```python
from build123d import *

# Parameters (mm, degrees)
SKETCH1_W           = 20
SKETCH1_H           = 20
BOSS_EXTRUDE1_DEPTH = 20
SKETCH2_W           = 20
SKETCH2_H           = 40.2
BOSS_EXTRUDE2_DEPTH = 64.7
SKETCH3_W           = 40.9
SKETCH3_H           = 20.8
CUT_EXTRUDE1_DEPTH  = 90.320210479
SKETCH4_W           = 11.9
SKETCH4_H           = 40.2
CUT_EXTRUDE2_DEPTH  = 90.320210479
SKETCH5_R           = 2.35
CUT_EXTRUDE3_DEPTH  = 10
SKETCH6_R           = 2.35
CUT_EXTRUDE4_DEPTH  = 10
CHAMFER1_SIZE       = 1
SKETCH7_W           = 20
SKETCH7_H           = 10.1
BOSS_EXTRUDE4_DEPTH = 4.7
SKETCH9_W           = 20
SKETCH9_H           = 20
BOSS_EXTRUDE5_DEPTH = 24.7
SKETCH10_R          = 3
CUT_EXTRUDE5_DEPTH  = 2
FILLET1_R           = 3.23
SKETCH11_W          = 20.2
SKETCH11_H          = 20.2
SKETCH11_W_2        = 20
SKETCH11_H_2        = 20
BOSS_EXTRUDE6_DEPTH = 40
SKETCH12_R          = 3.35
BOSS_EXTRUDE7_DEPTH = 0.1
BOSS_EXTRUDE8_DEPTH = 0.1


with BuildPart() as part:
    # Sketch1 → Boss-Extrude1 (new body)
    with BuildSketch(Plane(origin=(0, 0, 0), x_dir=(0, 0, -1), z_dir=(1, 0, 0))):
        Rectangle(SKETCH1_W, SKETCH1_H)
    extrude(amount=BOSS_EXTRUDE1_DEPTH)

    # Sketch2 → Boss-Extrude2 (add)
    with BuildSketch(Plane(origin=(20, 0, 0), x_dir=(0, 0, -1), z_dir=(1, 0, 0))):
        Rectangle(SKETCH2_W, SKETCH2_H)
    extrude(amount=BOSS_EXTRUDE2_DEPTH)

    # Sketch3 → Cut-Extrude1 (cut, through all)
    with BuildSketch(Plane.XY.offset(10)):
        with Locations((52.35, 0)):
            Rectangle(SKETCH3_W, SKETCH3_H)
    extrude(amount=-CUT_EXTRUDE1_DEPTH, mode=Mode.SUBTRACT)

    # Sketch4 → Cut-Extrude2 (cut, through all)
    with BuildSketch(Plane.XY.offset(10)):
        with Locations((78.75, 0)):
            Rectangle(SKETCH4_W, SKETCH4_H)
    extrude(amount=-CUT_EXTRUDE2_DEPTH, mode=Mode.SUBTRACT)

    # Sketch5 → Cut-Extrude3 (cut)
    with BuildSketch(Plane.XY.offset(10)):
        with Locations((28.01, 4.9)):
            Circle(SKETCH5_R)
        with Locations(Location((28.01, -4.9, 0), (0, 0, 180))):
            Circle(SKETCH5_R)
    extrude(amount=-CUT_EXTRUDE3_DEPTH, mode=Mode.SUBTRACT)

    # Sketch6 → Cut-Extrude4 (cut)
    with BuildSketch(Plane(origin=(72.8, 0, 0), x_dir=(0, 0, -1), z_dir=(1, 0, 0))):
        with Locations((0, -15.25)):
            Circle(SKETCH6_R)
        with Locations(Location((0, 15.25, 0), (0, 0, 180))):
            Circle(SKETCH6_R)
    extrude(amount=-CUT_EXTRUDE4_DEPTH, mode=Mode.SUBTRACT)

    # Chamfer1
    chamfer1_edges = [part.edges().sort_by_distance(p)[0] for p in [
        (25.66, 4.9, 10),
        (30.36, -4.9, 10),
        (72.8, -15.25, 2.35),
        (72.8, 15.25, -2.35),
    ]]
    chamfer(chamfer1_edges, length=CHAMFER1_SIZE)

    # Sketch7 → Boss-Extrude4 (add)
    with BuildSketch(Plane.ZY.offset(-20)):
        with Locations((0, 15.05)):
            Rectangle(SKETCH7_W, SKETCH7_H)
        with Locations((0, -15.05)):
            Rectangle(SKETCH7_W, SKETCH7_H)
    extrude(amount=BOSS_EXTRUDE4_DEPTH)

    # Sketch9 → Boss-Extrude5 (add)
    with BuildSketch(Plane.ZY):
        Rectangle(SKETCH9_W, SKETCH9_H)
    extrude(amount=BOSS_EXTRUDE5_DEPTH)

    # Sketch10 → Cut-Extrude5 (cut)
    with BuildSketch(Plane.ZY.offset(24.7)):
        Circle(SKETCH10_R)
    extrude(amount=-CUT_EXTRUDE5_DEPTH, mode=Mode.SUBTRACT)

    # Fillet1
    # the kernel refuses this fillet: 3.23 mm, written as the material it adds along each edge
    with BuildSketch(Plane(origin=(-22.7, 0, 0), x_dir=(0, 0, 1), z_dir=(0, -1, 0))) as fillet1_piece_1:
        with BuildLine():
            CenterArc((0.013363095, 3.23), FILLET1_R, 270, 67.616447755)
            Line((0.013363095, 0), (0.013363095, -0.0646))
            Line((0.013363095, -0.0646), (3, -0.0646))
            Line((3, -0.0646), (3.0646, 0))
            ThreePointArc((3.0646, 0), (3.0646, 1), (3.059732738, 1.9754))
            Line((3.059732738, 1.9754), (3, 2))
        make_face()
    revolve(axis=Axis((-22.7, 0, 0), (-1, 0, 0)))

    # Sketch11 → Boss-Extrude6 (add)
    with BuildSketch(Plane.ZY.offset(24.7)):
        Rectangle(SKETCH11_W, SKETCH11_H)
        Rectangle(SKETCH11_W_2, SKETCH11_H_2, mode=Mode.SUBTRACT)
    extrude(amount=-BOSS_EXTRUDE6_DEPTH)

    # Sketch12 → Boss-Extrude7 (add)
    with BuildSketch(Plane.XY.offset(10)):
        Polygon((72.8, 20.1), (15.3, 20.1), (15.3, -20.1), (72.8, -20.1), (72.8, -10.4), (31.9, -10.4), (31.9, 10.4), (72.8, 10.4), align=None)
        with Locations(Location((28.01, 4.9, 0), (0, 0, 180))):
            Circle(SKETCH12_R, mode=Mode.SUBTRACT)
        with Locations(Location((28.01, -4.9, 0), (0, 0, 180))):
            Circle(SKETCH12_R, mode=Mode.SUBTRACT)
    extrude(amount=BOSS_EXTRUDE7_DEPTH)

    # Sketch13 → Boss-Extrude8 (add)
    with BuildSketch(Plane(origin=(0, 0, -10), x_dir=(-1, 0, 0), z_dir=(0, 0, -1))):
        Polygon((-72.8, -20.1), (-15.3, -20.1), (-15.3, 20.1), (-72.8, 20.1), (-72.8, 10.4), (-31.9, 10.4), (-31.9, -10.4), (-72.8, -10.4), align=None)
    extrude(amount=BOSS_EXTRUDE8_DEPTH)


solid = part.part
```
Input: part model. Units: mm. Frame: model coordinates. A direction names the side the tool comes from. Give positions to 0.01 mm unless a question says otherwise; leave off trailing zeros. Write each loop counter-clockwise with the first axis right and the second up, starting at its lowest first coordinate (ties: lowest second). Pieces come first, ordered by that corner, then holes. Notation, with made-up numbers: (7, -12) - (61, -12) arc R11 cw to (61, -3) - close; hole circle Ø6 at (16.25, 12). An arc over 180 degrees is marked (long way). Write item = value, one per line. Start each with the question number.
1. Access query for faces 1 (the flat face through (62.8, 15, 0)), 2 (the flat face through (53, 10.4, 0)), 3 (the flat face through (28, -5, 0)), 4 (the flat face through (-5, 10.1, 0)). Directions: +Z, -Z, +X, -X, +Y, -Y. A direction counts if a zero-diameter tool reaches every point of the face in a straight line with its end or side. Return the directions, or none.
2. Section query D-D, the plane x = 28.01. Output: boundary loops of the cut face in (y, z).
3. Mould query, pull axis X, two halves, no side actions, for faces 5 (the flat face through (31.9, 0, 0)), 6 (the cylindrical face through (67.363, -17.544, 0.509)), 7 (the cylindrical face through (29.875, -3.47, 4.563)). Classes: released by +X, released by -X, zero draft, split by the parting line, or undercut.
4. Section query C-C, the plane z = -6. Output: boundary loops of the cut face in (x, y).
5. Section query A-A, the plane x = 60. Output: boundary loops of the cut face in (y, z).
6. Section query B-B, the plane y = -4.9. Output: boundary loops of the cut face in (x, z), then the cut area to 3 significant figures.
7. First-contact query: pin 1 Ø3 at (y, z) = (15.25, 0) entering from -X; pin 2 Ø10 at (x, z) = (2, 2.5) entering from +Y; pin 3 Ø1.4 at (y, z) = (16, 1) entering from +X; pin 4 Ø1.5 at (x, y) = (-12.5, 12.5) entering from -Z. Flat tips, straight axial feed; report the tip coordinate or a pass-through.
8. Ray query, L1, parallel to Y at x = 67.75, z = 0; L2, parallel to Y at x = 28.01, z = 2.75; L3, parallel to Y at x = 63, z = 8. Return the intervals inside material, ascending.
Check sheet entries:
q1.face_1 = +X
q1.face_2 = +Z, -Z, +X
q1.face_3 = +Z
q1.face_4 = +Z, -Z, -X, +Y
q2.outline = (-20.1, -10.1) - (20.1, -10.1) - (20.1, 10.1) - (8.25, 10.1) - (8.25, 10) - (7.25, 9) - (7.25, 0) - (2.55, 0) - (2.55, 9) - (1.55, 10) - (1.55, 10.1) - (-1.55, 10.1) - (-1.55, 10) - (-2.55, 9) - (-2.55, 0) - (-7.25, 0) - (-7.25, 9) - (-8.25, 10) - (-8.25, 10.1) - (-20.1, 10.1) - close
q3.face_5 = released by +X
q3.face_6 = zero draft
q3.face_7 = undercut
q4.outline = (-24.7, -10.1) - (15.3, -10.1) - (15.3, -20.1) - (72.8, -20.1) - (72.8, -10.4) - (31.9, -10.4) - (31.9, 10.4) - (72.8, 10.4) - (72.8, 20.1) - (15.3, 20.1) - (15.3, 10.1) - (-24.7, 10.1) - close
q5.outline = (-20.1, -10.1) - (-10.4, -10.1) - (-10.4, 10.1) - (-20.1, 10.1) - close; (10.4, -10.1) - (20.1, -10.1) - (20.1, 10.1) - (10.4, 10.1) - close
q6.outline = (-24.7, -10.1) - (31.9, -10.1) - (31.9, 10.1) - (31.36, 10.1) - (31.36, 10) - (30.36, 9) - (30.36, 0) - (25.66, 0) - (25.66, 9) - (24.66, 10) - (24.66, 10.1) - (-24.7, 10.1) - close
q6.area = 1,090 mm2
q7.pin_1 = 15.3
q7.pin_2 = 10.1
q7.pin_3 = 62.8
q7.pin_4 = through
q8.L1 = -20.1 to -17.6, -12.9 to -10.4, 10.4 to 12.9, 17.6 to 20.1
q8.L2 = -20.1 to -7.25, -2.55 to 2.55, 7.25 to 20.1
q8.L3 = -20.1 to -10.4, 10.4 to 20.1
